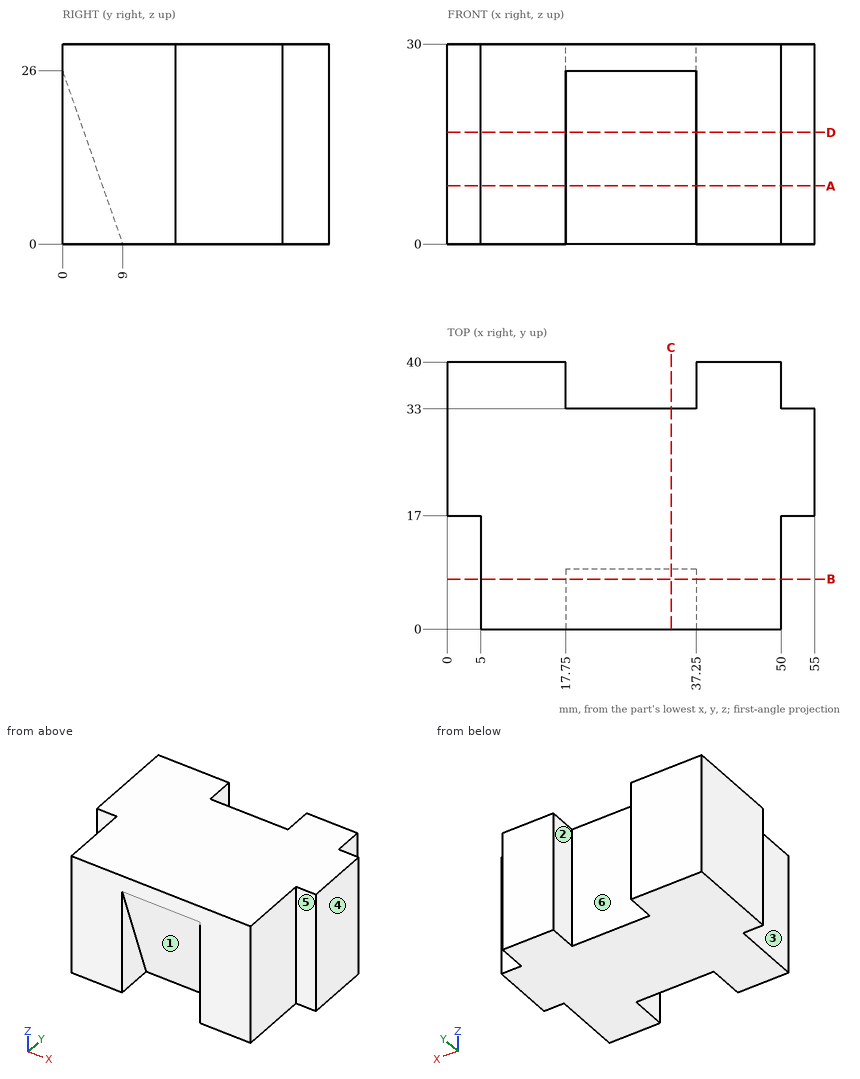
Could you check a few things on this drawing? It's one solid part, dimensions in mm from its lowest x, y, z. A direction names the side the tool comes from. Coordinates: 2 decimals unless noted, no trailing zeros. Write each loop counter-clockwise with the first axis right and the second up, starting at its lowest first coordinate (ties: lowest second). Pieces come first, ordered by that corner, then holes.
Q1. Please list where these lines run through material, in increasing order: L1, parallel to Y at x = 25, z = 27.5; L2, parallel to X at y = 33.5, z = 24; L3, parallel to X at y = 9, z = 25.
Results found:
L1: y = 0 to 33
L2: x = 0 to 17.75, 37.25 to 50
L3: x = 5 to 50
Q2. Which directions (+Z, -Z, +X, -X, +Y, -Y) give clear straight access to the entire face, cutting with the end or side of a thin tool? Please do the marked faces 1, 2 and 3.
Results found:
face 1: -Z, -Y
face 2: +Z, -Z, +Y
face 3: +Z, -Z, -X, -Y
Q3. Imagine slicing it at C-C, the plane x = 33.5. List the corners of the cut face in (y, z) for me.
Results found:
outline: (0, 26) - (9, 0) - (33, 0) - (33, 30) - (0, 30) - close
Q4. Imagine slicing it at D-D, the plane z = 16.75. List the corners of the cut face in (x, y) for me.
Results found:
outline: (0, 17) - (5, 17) - (5, 0) - (17.75, 0) - (17.75, 3.2) - (37.25, 3.2) - (37.25, 0) - (50, 0) - (50, 17) - (55, 17) - (55, 33) - (50, 33) - (50, 40) - (37.25, 40) - (37.25, 33) - (17.75, 33) - (17.75, 40) - (0, 40) - close
Q5. Imagine slicing it at A-A, the plane z = 8.75. List the corners of the cut face in (x, y) for me.
Results found:
outline: (0, 17) - (5, 17) - (5, 0) - (17.75, 0) - (17.75, 5.97) - (37.25, 5.97) - (37.25, 0) - (50, 0) - (50, 17) - (55, 17) - (55, 33) - (50, 33) - (50, 40) - (37.25, 40) - (37.25, 33) - (17.75, 33) - (17.75, 40) - (0, 40) - close
Q6. For P1, Ø8.5, axis at y = 10, z = 8.5, coming from the -X side; P2, Ø3.5, axis at y = 36, z = 7.5, coming from the +X side; P3, Ø1.5, axis at x = 52, z = 13.5, coming from the -Y side, each with a flat end and sliding along its axis, tell me the tip position at first contact or that it passes through.
Results found:
P1: stops at x = 5
P2: stops at x = 50
P3: stops at y = 17
Q7. Imagine slicing it at B-B, the plane y = 7.5. List the corners of the cut face in (x, z) for me.
Results found:
outline: (5, 0) - (17.75, 0) - (17.75, 4.33) - (37.25, 4.33) - (37.25, 0) - (50, 0) - (50, 30) - (5, 30) - close
Q8. If we mould it in two halves opening along X, with no side actions, what happens to the marked faces 4, 5 and 6? For each: +X half, -X half, draft (parallel to the pull), parting line (faces both ways), or undercut.
Results found:
face 4: +X half
face 5: draft
face 6: undercut
